Check sheet for the modelled part. Datum: model origin and axes. Units: mm. A direction names the side the tool comes from. Round coordinates to 2 decimals unless told otherwise and drop trailing zeros. Write each loop counter-clockwise with the first axis right and the second up, starting at its lowest first coordinate (ties: lowest second). Pieces come first, ordered by that corner, then holes.
from build123d import *

# Parameters (mm, degrees)
SKETCH1_R           = 23.5
BOSS_EXTRUDE1_DEPTH = 7
SKETCH2_R           = 1.5
BOSS_EXTRUDE2_DEPTH = 3
FILLET1_R           = 2


with BuildPart() as part:
    # Sketch1 → Boss-Extrude1 (new body)
    with BuildSketch(Plane(origin=(0, 0, 0), x_dir=(1, 0, 0), z_dir=(0, 1, 0))):
        with Locations(Location((0, 0, 0), (0, 0, 270))):
            Circle(SKETCH1_R)
    extrude(amount=BOSS_EXTRUDE1_DEPTH)

    # Sketch2 → Boss-Extrude2 (add)
    with BuildSketch(Plane.XY.offset(23.5)):
        with BuildLine():
            Line((-25, 0), (25, 0))
            ThreePointArc((25, 0), (28.5, 3.5), (25, 7))
            Line((25, 7), (-25, 7))
            ThreePointArc((-25, 7), (-28.5, 3.5), (-25, 0))
        make_face()
        with Locations((25, 3.5)):
            Circle(SKETCH2_R, mode=Mode.SUBTRACT)
        with Locations((-25, 3.5)):
            Circle(SKETCH2_R, mode=Mode.SUBTRACT)
    extrude(amount=-BOSS_EXTRUDE2_DEPTH)

    # Fillet1
    fillet1_edges = [part.edges().sort_by_distance(p)[0] for p in [
        (-11.489125293, 3.5, 20.5),
        (11.489125293, 3.5, 20.5),
    ]]
    fillet(fillet1_edges, radius=FILLET1_R)


solid = part.part
1. Sectioned sample at C-C, the plane z = 0. Enter the section's corners in (x, y).
2. Go/stop test with flat-tipped pins: pin 1 (1 mm diameter, centred on y = 3, z = 3.5, fed in from -X); pin 2 (2.5 mm diameter, centred on x = 25, y = 3.5, fed in from +Z); pin 3 (2 mm diameter, centred on x = -22.5, y = 2.5, fed in from -Z). Record where each tip stops, or that it passes through.
3. Sectioned sample at D-D, the plane x = -12.5. Enter the section's corners in (y, z), plus the area to 3 significant figures.
4. Set-up check for faces 5 (the flat face through (23, 4, 20.5)), 6 (the cylindrical face through (0.784, 3.451, -23.487)): record each of +Z, -Z, +X, -X, +Y, -Y from which the full face is reachable in a straight line by a thin tool's end or side.
5. Sectioned sample at A-A, the plane x = -22. Enter the section's corners in (y, z), plus the area to 3 significant figures.
6. Sectioned sample at B-B, the plane y = 3.5. Enter the section's corners in (x, z), plus the area to 3 significant figures.
7. Scan lines: line 1 along Y through (x, z) = (-25, 22); line 2 along Z through (x, y) = (26.5, 6.25); line 3 along Z through (x, y) = (-21.5, 1.25). Record each from-to range of solid material in increasing order.
8. Release check for a two-part mould opening along Z. For faces 1 (the flat face through (-23, 4, 20.5)), 2 (the cylindrical face through (-15.68, 3.45, 19.21)), 3 (the flat face through (0, 4, 23.5)), 4 (the cylindrical face through (-26.5, 3.57, 22.02)) record: released by +Z, released by -Z, zero draft, split by the parting line, or undercut.
Computed values:
1. outline: (-23.5, 0) - (23.5, 0) - (23.5, 7) - (-23.5, 7) - close
2. pin 1: stops at x = -23.31
2. pin 2: passes through
2. pin 3: stops at z = -9.49
3. outline: (0, -19.9) - (7, -19.9) - (7, 23.5) - (0, 23.5) - close
3. area: 304 mm2
4. face 5: +X, +Y, -Y
4. face 6: +Y, -Y
5. outline: (0, -8.26) - (7, -8.26) - (7, 8.26) - (0, 8.26) - close; (0, 20.5) - (7, 20.5) - (7, 23.5) - (0, 23.5) - close
5. area: 137 mm2
6. outline: (-28.5, 20.5) - (-26.5, 20.5) - (-26.5, 23.5) - (-28.5, 23.5) - close; (-23.5, 20.5) - (-17.55, 20.5) arc R2 cw to (-16.17, 17.05) arc R23.5 ccw (long way) to (16.17, 17.05) arc R2 cw to (17.55, 20.5) - (23.5, 20.5) - (23.5, 23.5) - (-23.5, 23.5) - close; (26.5, 20.5) - (28.5, 20.5) - (28.5, 23.5) - (26.5, 23.5) - close
6. area: 1,850 mm2
7. line 1: y = 0 to 2, 5 to 7
7. line 2: z = 20.5 to 23.5
7. line 3: z = -9.49 to 9.49, 20.5 to 23.5
8. face 1: undercut
8. face 2: undercut
8. face 3: released by +Z
8. face 4: zero draft
